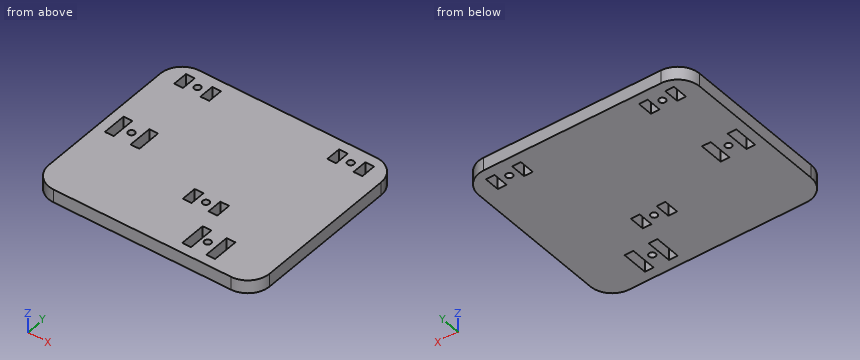
Autodesk Fusion 360 part; units mm, degrees
sketch "Sketch1" plane through (0, 0, 0) normal (0, 0, 1) x (1, 0, 0)
  line L0 (10, 0) -> (91, 0)
  line L1 (101, 10) -> (101, 75.843)
  line L2 (91, 85.843) -> (10, 85.843)
  line L3 (0, 75.843) -> (0, 10)
  line L4 (8, 80.843) -> (23, 80.843)
  line L5 (23, 80.843) -> (23, 74.843)
  line L6 (23, 74.843) -> (8, 74.843)
  line L7 (8, 74.843) -> (8, 80.843)
  line L8 (23, 80.843) -> (78, 80.843)
  line L9 (78, 80.843) -> (93, 80.843)
  line L10 (93, 80.843) -> (93, 74.843)
  line L11 (93, 74.843) -> (78, 74.843)
  line L12 (78, 74.843) -> (78, 80.843)
  line L13 (11, 80.843) -> (11, 74.843)
  line L14 (20, 80.843) -> (20, 74.843)
  line L15 (90, 80.843) -> (90, 74.843)
  line L16 (81, 74.843) -> (81, 80.843)
  line L17 (50.5, 85.843) -> (50.5, 80.843)
  line L18 (5, 47.843) -> (19.74, 47.843)
  line L19 (19.74, 47.843) -> (19.74, 37.843)
  line L20 (19.74, 37.843) -> (5, 37.843)
  line L21 (5, 37.843) -> (5, 47.843)
  line L22 (5, 47.843) -> (8, 47.843)
  line L23 (8, 47.843) -> (8, 37.843)
  line L24 (8, 37.843) -> (5, 37.843)
  line L25 (5, 37.843) -> (5, 47.843)
  line L26 (19.74, 37.843) -> (16.74, 37.843)
  line L27 (16.74, 37.843) -> (16.74, 47.843)
  line L28 (16.74, 47.843) -> (19.74, 47.843)
  line L29 (19.74, 47.843) -> (19.74, 37.843)
  line L30 (50.557, 31) -> (65.297, 31)
  line L31 (65.297, 31) -> (65.297, 25)
  line L32 (65.297, 25) -> (50.557, 25)
  line L33 (50.557, 25) -> (50.557, 31)
  line L34 (50.557, 31) -> (53.557, 31)
  line L35 (53.557, 31) -> (53.557, 25)
  line L36 (53.557, 25) -> (50.557, 25)
  line L37 (50.557, 25) -> (50.557, 31)
  line L38 (65.297, 25) -> (62.297, 25)
  line L39 (62.297, 25) -> (62.297, 31)
  line L40 (62.297, 31) -> (65.297, 31)
  line L41 (65.297, 31) -> (65.297, 25)
  line L42 (65.797, 16) -> (79.797, 16)
  line L43 (79.797, 16) -> (79.797, 5)
  line L44 (79.797, 5) -> (65.797, 5)
  line L45 (65.797, 5) -> (65.797, 16)
  line L46 (68.797, 16) -> (68.797, 5)
  line L47 (76.797, 5) -> (76.797, 16)
  arc A0 (10, 85.843) -> (0, 75.843) centre (10, 75.843) ccw
  arc A1 (101, 75.843) -> (91, 85.843) centre (91, 75.843) ccw
  arc A2 (0, 10) -> (10, 0) centre (10, 10) ccw
  arc A3 (91, 0) -> (101, 10) centre (91, 10) ccw
  line L48 (11, 77.843) -> (20, 77.843)
  line L49 (8, 42.843) -> (16.74, 42.843)
  line L50 (81, 77.843) -> (90, 77.843)
  line L51 (53.557, 28) -> (62.297, 28)
  line L52 (68.797, 10.5) -> (76.797, 10.5)
  circle A4 centre (72.297, 10.5) radius 1.5
  circle A5 centre (57.927, 28) radius 1.5
  circle A6 centre (12.37, 42.843) radius 1.5
  circle A7 centre (15.5, 77.843) radius 1.5
  circle A8 centre (85.5, 77.843) radius 1.5
  circle A9 centre (72.297, 10.5) radius 3.5
  dimension "d1" = 6
  dimension "d2" = 6
  dimension "d3" = 15
  dimension "d4" = 15
  dimension "d5" = 55
  dimension "d6" = 3
  dimension "d7" = 3
  dimension "d8" = 3
  dimension "d9" = 3
  dimension "d10" = 90
  dimension "d11" = 5
  dimension "d12" = 14.74
  dimension "d13" = 10
  dimension "d14" = 3
  dimension "d15" = 3
  dimension "d16" = 27
  dimension "d17" = 3
  dimension "d18" = 14.74
  dimension "d19" = 6
  dimension "d20" = 3
  dimension "d21" = 3
  dimension "d22" = 6.843
  dimension "d23" = 30.817
  dimension "d24" = 14
  dimension "d25" = 11
  dimension "d26" = 3
  dimension "d27" = 3
  dimension "d28" = 0.5
  dimension "d29" = 9
  dimension "d30" = 5
  dimension "d31" = 8
  dimension "d32" = 8
  dimension "d33" = 5
  dimension "d34" = 10
  dimension "d35" = 10
  dimension "d36" = 10
  dimension "d37" = 10
  dimension "d38" = 7
  dimension "d39" = 3
  dimension "d40" = 3
  dimension "d41" = 3
  dimension "d42" = 3
  dimension "d43" = 3
extrude "Extrude1" add sketch "Sketch1" along normal blind 6 contours L0 L1 L2 L3 A0 A1 A2 A3 | L4 L13 L14 L48 A7 | L9 L15 L16 L50 A8 | L6 L13 L14 L48 A7 | L11 L15 L16 L50 A8 | L18 L23 L27 L49 A6 | L20 L23 L27 L49 A6 | L30 L35 L39 L51 A5 | L32 L35 L39 L51 A5 | L42 L46 L47 L52 A9 | L44 L46 L47 L52 A9 | L52 A4 A9 | L52 A4 A9
sketch "Sketch2" plane through (0, 0, 6) normal (0, 0, 1) x (-1, 0, 0)
  line L0 (-8, -80.843) -> (-11, -80.843)
  line L1 (-11, -80.843) -> (-11, -74.843)
  line L2 (-11, -74.843) -> (-8, -74.843)
  line L3 (-8, -74.843) -> (-8, -80.843)
  line L4 (-16.74, -47.843) -> (-19.74, -47.843)
  line L5 (-19.74, -47.843) -> (-19.74, -37.843)
  line L6 (-19.74, -37.843) -> (-16.74, -37.843)
  line L7 (-16.74, -37.843) -> (-16.74, -47.843)
  line L8 (-65.797, -16) -> (-68.797, -16)
  line L9 (-68.797, -16) -> (-68.797, -5)
  line L10 (-68.797, -5) -> (-65.797, -5)
  line L11 (-65.797, -5) -> (-65.797, -16)
  circle A0 centre (-57.927, -28) radius 1.5
  line L12 (-81, -74.843) -> (-78, -74.843)
  line L13 (-78, -74.843) -> (-78, -80.843)
  line L14 (-78, -80.843) -> (-81, -80.843)
  line L15 (-81, -80.843) -> (-81, -74.843)
  circle A1 centre (-85.5, -77.843) radius 1.5
  line L16 (-90, -80.843) -> (-93, -80.843)
  line L17 (-93, -80.843) -> (-93, -74.843)
  line L18 (-93, -74.843) -> (-90, -74.843)
  line L19 (-90, -74.843) -> (-90, -80.843)
  circle A2 centre (-15.5, -77.843) radius 1.5
  line L20 (-20, -80.843) -> (-23, -80.843)
  line L21 (-23, -80.843) -> (-23, -74.843)
  line L22 (-23, -74.843) -> (-20, -74.843)
  line L23 (-20, -74.843) -> (-20, -80.843)
  line L24 (-53.557, -25) -> (-50.557, -25)
  line L25 (-50.557, -25) -> (-50.557, -31)
  line L26 (-50.557, -31) -> (-53.557, -31)
  line L27 (-53.557, -31) -> (-53.557, -25)
  line L28 (-8, -37.843) -> (-5, -37.843)
  line L29 (-5, -37.843) -> (-5, -47.843)
  line L30 (-5, -47.843) -> (-8, -47.843)
  line L31 (-8, -47.843) -> (-8, -37.843)
  circle A3 centre (-72.297, -10.5) radius 1.5
  circle A4 centre (-12.37, -42.843) radius 1.5
  line L32 (-62.297, -31) -> (-65.297, -31)
  line L33 (-65.297, -31) -> (-65.297, -25)
  line L34 (-65.297, -25) -> (-62.297, -25)
  line L35 (-62.297, -25) -> (-62.297, -31)
  line L36 (-79.797, -5) -> (-76.797, -5)
  line L37 (-76.797, -5) -> (-76.797, -16)
  line L38 (-76.797, -16) -> (-79.797, -16)
  line L39 (-79.797, -16) -> (-79.797, -5)
  arc A5 (-91, 0) -> (-101, -10) centre (-91, -10) ccw
  line L40 (-101, -10) -> (-101, -75.843)
  arc A6 (-101, -75.843) -> (-91, -85.843) centre (-91, -75.843) ccw
  line L41 (-91, -85.843) -> (-10, -85.843)
  arc A7 (-10, -85.843) -> (0, -75.843) centre (-10, -75.843) ccw
  line L42 (0, -75.843) -> (0, -10)
  arc A8 (0, -10) -> (-10, 0) centre (-10, -10) ccw
  line L43 (-10, 0) -> (-91, 0)
  line L44 (-7.5, -74.343) -> (-7.5, -81.343)
  line L45 (-7.5, -81.343) -> (-11.5, -81.343)
  line L46 (-11.5, -81.343) -> (-11.5, -74.343)
  line L47 (-11.5, -74.343) -> (-7.5, -74.343)
  line L48 (-23.5, -74.343) -> (-19.5, -74.343)
  line L49 (-19.5, -74.343) -> (-19.5, -81.343)
  line L50 (-19.5, -81.343) -> (-23.5, -81.343)
  line L51 (-23.5, -81.343) -> (-23.5, -74.343)
  line L52 (-81.5, -74.343) -> (-77.5, -74.343)
  line L53 (-77.5, -74.343) -> (-77.5, -81.343)
  line L54 (-77.5, -81.343) -> (-81.5, -81.343)
  line L55 (-81.5, -81.343) -> (-81.5, -74.343)
  line L56 (-93.5, -81.343) -> (-93.5, -74.343)
  line L57 (-93.5, -74.343) -> (-89.5, -74.343)
  line L58 (-89.5, -74.343) -> (-89.5, -81.343)
  line L59 (-89.5, -81.343) -> (-93.5, -81.343)
  line L60 (-4.5, -37.343) -> (-4.5, -48.343)
  line L61 (-4.5, -48.343) -> (-8.5, -48.343)
  line L62 (-8.5, -48.343) -> (-8.5, -37.343)
  line L63 (-8.5, -37.343) -> (-4.5, -37.343)
  line L64 (-20.24, -37.343) -> (-16.24, -37.343)
  line L65 (-16.24, -37.343) -> (-16.24, -48.343)
  line L66 (-16.24, -48.343) -> (-20.24, -48.343)
  line L67 (-20.24, -48.343) -> (-20.24, -37.343)
  line L68 (-50.057, -31.5) -> (-54.057, -31.5)
  line L69 (-54.057, -31.5) -> (-54.057, -24.5)
  line L70 (-54.057, -24.5) -> (-50.057, -24.5)
  line L71 (-50.057, -24.5) -> (-50.057, -31.5)
  line L72 (-61.797, -31.5) -> (-65.797, -31.5)
  line L73 (-65.797, -31.5) -> (-65.797, -24.5)
  line L74 (-65.797, -24.5) -> (-61.797, -24.5)
  line L75 (-61.797, -24.5) -> (-61.797, -31.5)
  line L76 (-69.297, -4.5) -> (-65.297, -4.5)
  line L77 (-65.297, -4.5) -> (-65.297, -16.5)
  line L78 (-65.297, -16.5) -> (-69.297, -16.5)
  line L79 (-69.297, -16.5) -> (-69.297, -4.5)
  line L80 (-80.297, -4.5) -> (-76.297, -4.5)
  line L81 (-76.297, -4.5) -> (-76.297, -16.5)
  line L82 (-76.297, -16.5) -> (-80.297, -16.5)
  line L83 (-80.297, -16.5) -> (-80.297, -4.5)
  dimension "d46" = -0.5
  dimension "d47" = -0.5
  dimension "d48" = -0.5
  dimension "d49" = -0.5
  dimension "d50" = -0.5
  dimension "d51" = -0.5
  dimension "d52" = -0.5
  dimension "d53" = -0.5
  dimension "d54" = -0.5
  dimension "d55" = -0.5
extrude "Extrude2" cut sketch "Sketch2" against normal blind 10 contours L44 L45 L46 L47 | L48 L49 L50 L51 | L52 L53 L54 L55 | L56 L57 L58 L59 | L60 L61 L62 L63 | L64 L65 L66 L67 | L68 L69 L70 L71 | L72 L73 L74 L75 | L76 L77 L78 L79 | L80 L81 L82 L83
Source: CAD feature listing. Evaluate the final solid. Frame: model axes, mm. Round coordinates to 2 decimals unless told otherwise and drop trailing zeros. Order: outer loops, then holes, each group sorted by start corner. A loop starts at its lowest first (then second) coordinate and runs counter-clockwise, first axis right, second up. Notation, with made-up numbers: (-19.5, 40) - (-6.5, 40) arc R11 cw to (-6.5, 48) - close; hole circle Ø10 at (41.5, 32.25). An arc over 180 degrees is marked (long way). Use a Markdown table: item, result. Add a question column.
1. Line query: probe 1 along X at (y, z) = (43, 5.45); probe 2 along Y at (x, z) = (78, 4.35); probe 3 along X at (y, z) = (10.5, 2.4). Output: solid intervals per line, ascending.
2. Section query A-A (x = 85.5). Return the cut outline in (y, z).
3. Section query B-B (y = 28). Return the cut outline in (x, z), then the cut area to 3 significant figures.
4. Section query C-C (z = 3.7). Give the number of separate pieces and of enclosed holes in the cut face, then the cut area to 3 significant figures.
5. First-contact query: pin 1 (3 mm diameter, centred on y = 78.5, z = 2.5, fed in from +X); pin 2 (1.2 mm diameter, centred on x = 6, z = 2.5, fed in from +Y); pin 3 (3 mm diameter, centred on y = 79.5, z = 3, fed in from -X). Flat tips, straight axial feed; report the tip coordinate or a pass-through.
Derived:
| question | item | result |
|---|---|---|
| 1 | probe 1 | 0 to 4.5, 8.5 to 10.88, 13.86 to 16.24, 20.24 to 101 |
| 1 | probe 2 | 0 to 4.5, 16.5 to 74.34, 81.34 to 85.84 |
| 1 | probe 3 | 0 to 65.3, 69.3 to 70.8, 73.8 to 76.3, 80.3 to 101 |
| 2 | outline | (0, 0) - (76.34, 0) - (76.34, 6) - (0, 6) - close; (79.34, 0) - (85.84, 0) - (85.84, 6) - (79.34, 6) - close |
| 3 | outline | (0, 0) - (50.06, 0) - (50.06, 6) - (0, 6) - close; (54.06, 0) - (56.43, 0) - (56.43, 6) - (54.06, 6) - close; (59.43, 0) - (61.8, 0) - (61.8, 6) - (59.43, 6) - close; (65.8, 0) - (101, 0) - (101, 6) - (65.8, 6) - close |
| 3 | area | 540 mm2 |
| 4 | separate pieces | 1 |
| 4 | enclosed holes | 15 |
| 4 | area | 8,200 mm2 |
| 5 | pin 1 | x = 100.93 |
| 5 | pin 2 | y = 85.25 |
| 5 | pin 3 | x = 0.24 |
